from build123d import *

# Parameters (mm, degrees)
SKETCH1_W           = 20
SKETCH1_H           = 20
SKETCH1_W_2         = 16
SKETCH1_H_2         = 16
BOSS_EXTRUDE1_DEPTH = 1300
SKETCH2_W           = 20
SKETCH2_H           = 20
BOSS_EXTRUDE2_DEPTH = 1
SKETCH3_W           = 20
SKETCH3_H           = 20
BOSS_EXTRUDE3_DEPTH = 1


with BuildPart() as part:
    # Sketch1 → Boss-Extrude1 (new body)
    with BuildSketch(Plane(origin=(0, 0, 0), x_dir=(1, 0, 0), z_dir=(0, 1, 0))):
        Rectangle(SKETCH1_W, SKETCH1_H)
        Rectangle(SKETCH1_W_2, SKETCH1_H_2, mode=Mode.SUBTRACT)
    extrude(amount=BOSS_EXTRUDE1_DEPTH)

    # Sketch2 → Boss-Extrude2 (add)
    with BuildSketch(Plane(origin=(0, 1300, 0), x_dir=(1, 0, 0), z_dir=(0, 1, 0))):
        Rectangle(SKETCH2_W, SKETCH2_H)
    extrude(amount=BOSS_EXTRUDE2_DEPTH)

    # Sketch3 → Boss-Extrude3 (add)
    with BuildSketch(Plane.XZ):
        Rectangle(SKETCH3_W, SKETCH3_H)
    extrude(amount=BOSS_EXTRUDE3_DEPTH)


solid = part.part
Geometry check sheet. Reference: the model listing, model coordinates, mm. Round coordinates to 2 decimals unless told otherwise and drop trailing zeros. Loops run counter-clockwise (first coordinate to the right, second up) from the corner with the lowest first, then second, coordinate; pieces in that order, holes last. Notation, with made-up numbers: (22.5, -35) -> (75.5, -35) arc R25 cw to (75.5, -3) -> close; hole circle Ø4 at (-34, 49.25). An arc over 180 degrees is marked (long way). Answer as a JSON object with one key per item and string values. Group by question number.
Item 1: Cross-section at A-A, the plane x = 0.25. Record the cut outline in (y, z), plus the area to 3 significant figures.
Item 2: Cross-section at B-B, the plane y = 191. Record the cut outline in (x, z).
Item 3: Thickness scan on line 1 along Z through (x, y) = (-5, 465.5); line 2 along Y through (x, z) = (0.5, -2.75). Record the ranges inside material, lowest first.
Item 4: Release check for a two-part mould opening along Y. For faces 1 (the face through (0, 1301, 0)), 2 (the face through (0, 659, -10)), 3 (the face through (0, -1, 0)) record: pulls with the +Y half, pulls with the -Y half, needs draft (parallel to the pull), parting line crosses it, or undercut.
Determined:
{
 "1": {"outline": "(-1, -10) -> (1301, -10) -> (1301, 10) -> (-1, 10) -> close; hole (0, -8) -> (1300, -8) -> (1300, 8) -> (0, 8) -> close", "area": "5,240 mm²"},
 "2": {"outline": "(-10, -10) -> (10, -10) -> (10, 10) -> (-10, 10) -> close; hole (-8, -8) -> (8, -8) -> (8, 8) -> (-8, 8) -> close"},
 "3": {"line 1": "z = -10 to -8, 8 to 10", "line 2": "y = -1 to 0, 1300 to 1301"},
 "4": {"face 1": "pulls with the +Y half", "face 2": "needs draft", "face 3": "pulls with the -Y half"}
}
